Build history of the part. All positions in model axes, mm. Coordinates: 2 decimals unless noted, no trailing zeros. Order: outer loops, then holes, each group sorted by start corner. A loop starts at its lowest first (then second) coordinate and runs counter-clockwise, first axis right, second up. Notation, with made-up numbers: (-15, 28.25) - (16, 28.25) arc R16 cw to (16, 51.25) - close; hole circle Ø9 at (67.25, 17). An arc over 180 degrees is marked (long way). Write each question's results on one line, items separated by ' | '.
from build123d import *

# Parameters (mm, degrees)
F0_W     = 76.2
F0_H     = 114.3
F0_R     = 3.2639
F0_R_2   = 4.1021
F1_DEPTH = 6.35


with BuildPart() as f1:
    # F0 (on Front) → F1 (new body)
    with BuildSketch(Plane.XZ):
        with Locations((38.1, 57.15)):
            Rectangle(F0_W, F0_H)
        with Locations((19.05, 19.05)):
            Circle(F0_R, mode=Mode.SUBTRACT)
        with Locations((57.15, 19.05)):
            Circle(F0_R, mode=Mode.SUBTRACT)
        with Locations((19.05, 57.15)):
            Circle(F0_R, mode=Mode.SUBTRACT)
        with Locations((19.05, 95.25)):
            Circle(F0_R_2, mode=Mode.SUBTRACT)
        with Locations((57.15, 57.15)):
            Circle(F0_R, mode=Mode.SUBTRACT)
        with Locations((38.1, 95.25)):
            Circle(F0_R, mode=Mode.SUBTRACT)
        with Locations((57.15, 95.25)):
            Circle(F0_R_2, mode=Mode.SUBTRACT)
    extrude(amount=F1_DEPTH)


solid = f1.part
1. Drop a flat-ended pin along its axis: pin 1 Ø7.5 at (x, z) = (19.05, 95.25) entering from +Y. Give the stop position or say it passes through.
Solved:
pin 1: passes through
2. Probe line 1 (Z direction, x = 57.15, y = -3); line 2 (X direction, y = -4.5, z = 95); line 3 (Z direction, x = 59, y = -5.5). List the from-to ranges inside material, lowest first.
Solved:
line 1: z = 0 to 15.79, 22.31 to 53.89, 60.41 to 91.15, 99.35 to 114.3 | line 2: x = 0 to 14.96, 23.14 to 34.85, 41.35 to 53.06, 61.24 to 76.2 | line 3: z = 0 to 16.36, 21.74 to 54.46, 59.84 to 91.59, 98.91 to 114.3
3. Band-saw the part on C-C on z = 57.15. Give the cut face in (x, y), then the cut area to 3 significant figures.
Solved:
outline: (0, -6.35) - (15.79, -6.35) - (15.79, 0) - (0, 0) - close; (22.31, -6.35) - (53.89, -6.35) - (53.89, 0) - (22.31, 0) - close; (60.41, -6.35) - (76.2, -6.35) - (76.2, 0) - (60.41, 0) - close | area: 401 mm2
4. Two-plate mould, pull along X, no slides. Class faces 1 (the face through (54.56, -3.131, 55.164)), 2 (the face through (56.616, -3.131, 99.317)), 3 (the face through (0, -3, 56)), 4 (the face through (76.2, -3, 56)): +X half, -X half, draft (parallel to the pull), parting line (faces both ways), or undercut.
Solved:
face 1: undercut | face 2: undercut | face 3: -X half | face 4: +X half
5. Band-saw the part on A-A on x = 38.1. Give the cut face in (y, z), then the cut area to 3 significant figures.
Solved:
outline: (-6.35, 0) - (0, 0) - (0, 91.99) - (-6.35, 91.99) - close; (-6.35, 98.51) - (0, 98.51) - (0, 114.3) - (-6.35, 114.3) - close | area: 684 mm2
6. Band-saw the part on D-D on y = -1.75. Give the cut face in (x, z).
Solved:
outline: (0, 0) - (76.2, 0) - (76.2, 114.3) - (0, 114.3) - close; hole circle Ø8.2 at (19.05, 95.25); hole circle Ø6.53 at (19.05, 19.05); hole circle Ø6.53 at (19.05, 57.15); hole circle Ø6.53 at (38.1, 95.25); hole circle Ø8.2 at (57.15, 95.25); hole circle Ø6.53 at (57.15, 19.05); hole circle Ø6.53 at (57.15, 57.15)
7. Band-saw the part on B-B on x = 57.15. Give the cut face in (y, z), then the cut area to 3 significant figures.
Solved:
outline: (-6.35, 0) - (0, 0) - (0, 15.79) - (-6.35, 15.79) - close; (-6.35, 22.31) - (0, 22.31) - (0, 53.89) - (-6.35, 53.89) - close; (-6.35, 60.41) - (0, 60.41) - (0, 91.15) - (-6.35, 91.15) - close; (-6.35, 99.35) - (0, 99.35) - (0, 114.3) - (-6.35, 114.3) - close | area: 591 mm2
